from build123d import *

# Parameters (mm, degrees)
SKETCH1_R           = 2.667
BOSS_EXTRUDE1_DEPTH = 1.5875
SKETCH2_W           = 3.302
SKETCH2_H           = 18.796
CUT_EXTRUDE1_DEPTH  = 4.175


with BuildPart() as part:
    # Sketch1 → Boss-Extrude1 (new body, symmetric)
    with BuildSketch(Plane(origin=(0, 0, 0), x_dir=(0, 0, -1), z_dir=(1, 0, 0))):
        with BuildLine():
            Line((-98.171, 17.907), (94.615, 17.907))
            Line((94.615, 17.907), (94.615, 13.462))
            Line((94.615, 13.462), (98.171, 13.462))
            Line((98.171, 13.462), (98.171, 4.826))
            Line((98.171, 4.826), (94.615, 4.826))
            Line((94.615, 4.826), (94.615, 2.667))
            Line((94.615, 2.667), (89.535, 2.667))
            Line((89.535, 2.667), (89.535, 4.191))
            Line((89.535, 4.191), (83.947, 4.191))
            Line((83.947, 4.191), (83.947, 2.667))
            Line((83.947, 2.667), (76.073, 2.667))
            Line((76.073, 2.667), (76.073, -2.667))
            Line((76.073, -2.667), (83.947, -2.667))
            Line((83.947, -2.667), (83.947, -4.191))
            Line((83.947, -4.191), (89.535, -4.191))
            Line((89.535, -4.191), (89.535, -2.667))
            Line((89.535, -2.667), (94.615, -2.667))
            Line((94.615, -2.667), (94.615, -4.826))
            Line((94.615, -4.826), (98.171, -4.826))
            Line((98.171, -4.826), (98.171, -13.462))
            Line((98.171, -13.462), (94.615, -13.462))
            Line((94.615, -13.462), (94.615, -17.907))
            Line((94.615, -17.907), (-98.171, -17.907))
            Line((-98.171, -17.907), (-98.171, -6.477))
            Line((-98.171, -6.477), (-80.391, -6.477))
            ThreePointArc((-80.391, -6.477), (-73.914, 0), (-80.391, 6.477))
            Line((-80.391, 6.477), (-98.171, 6.477))
            Line((-98.171, 6.477), (-98.171, 17.907))
        make_face()
        with Locations((-63.881, 10.287)):
            Circle(SKETCH1_R, mode=Mode.SUBTRACT)
        with Locations((-63.881, -10.287)):
            Circle(SKETCH1_R, mode=Mode.SUBTRACT)
        with Locations((-44.831, 11.303)):
            Circle(SKETCH1_R, mode=Mode.SUBTRACT)
        with Locations((21.717, 11.303)):
            Circle(SKETCH1_R, mode=Mode.SUBTRACT)
        with Locations((88.265, 11.303)):
            Circle(SKETCH1_R, mode=Mode.SUBTRACT)
        with Locations((88.265, -11.303)):
            Circle(SKETCH1_R, mode=Mode.SUBTRACT)
        with Locations((21.717, -11.303)):
            Circle(SKETCH1_R, mode=Mode.SUBTRACT)
        with Locations((-44.831, -11.303)):
            Circle(SKETCH1_R, mode=Mode.SUBTRACT)
        with Locations((-9.144, 10.795)):
            Circle(SKETCH1_R, mode=Mode.SUBTRACT)
        with Locations((-32.258, 10.795)):
            Circle(SKETCH1_R, mode=Mode.SUBTRACT)
        with Locations((66.802, 10.795)):
            Circle(SKETCH1_R, mode=Mode.SUBTRACT)
        with Locations((43.688, 10.795)):
            Circle(SKETCH1_R, mode=Mode.SUBTRACT)
        with Locations((43.688, -10.795)):
            Circle(SKETCH1_R, mode=Mode.SUBTRACT)
        with Locations((66.802, -10.795)):
            Circle(SKETCH1_R, mode=Mode.SUBTRACT)
        with Locations((-32.258, -10.795)):
            Circle(SKETCH1_R, mode=Mode.SUBTRACT)
        with Locations((-9.144, -10.795)):
            Circle(SKETCH1_R, mode=Mode.SUBTRACT)
        with Locations((-20.701, 0)):
            Circle(SKETCH1_R, mode=Mode.SUBTRACT)
        with Locations((55.245, 0)):
            Circle(SKETCH1_R, mode=Mode.SUBTRACT)
    extrude(amount=BOSS_EXTRUDE1_DEPTH, both=True)

    # Sketch2 → Cut-Extrude1 (cut, through all)
    with BuildSketch(Plane(origin=(1.5875, 0, 0), x_dir=(0, 0, -1), z_dir=(1, 0, 0))):
        with Locations((-52.705, 8.509)):
            Rectangle(SKETCH2_W, SKETCH2_H)
    extrude(amount=-CUT_EXTRUDE1_DEPTH, mode=Mode.SUBTRACT)


solid = part.part
Geometry check sheet. Reference: the model listing, model coordinates, mm. A direction names the side the tool comes from. Round coordinates to 2 decimals unless told otherwise and drop trailing zeros.
Item 1: Access from +Z, -Z, +X, -X, +Y, -Y to the whole of each face (thin tool, end or side, straight path). Record for faces 4 (the flat face through (0, -6.477, 89)), 5 (the flat face through (0, 2.667, -92)), 6 (the flat face through (0, 13.462, -96)), 7 (the flat face through (0, 8, 51.054)).
Item 2: Cross-section at A-A on x = -0.15. Count the separate pieces of the cut face and the enclosed holes in it, then the cut area to 3 significant figures.
Item 3: Mould release check, pull along Y, two halves, no side actions. Record for faces 1 (the flat face through (0, 17.907, 77)), 2 (the cylindrical face through (0, 13.1, 46.8)), 3 (the flat face through (0, 8, 54.356)): pulls with the +Y half, pulls with the -Y half, needs draft (parallel to the pull), parting line crosses it, or undercut.
Item 4: Thickness scan on line 1 (Y direction, x = 0.3, z = -43.5); line 2 (Y direction, x = -0.7, z = -44); line 3 (Y direction, x = -1.1, z = 74.5). Record the ranges inside material, lowest first.
Item 5: Gauge pin test, flat ends, axial feed: pin 1 (4.5 mm diameter, centred on y = -10.795, z = -43.688, fed in from +X); pin 2 (1.7 mm diameter, centred on x = -0.5, y = -3.5, fed in from -Z) (3 decimals); pin 3 (1.6 mm diameter, centred on x = 0.5, z = -96, fed in from -Y). Record the tip position at first contact, or that the pin passes through.
Answer sheet:
1. face 4: +Z, +X, -X
1. face 5: -Z, +X, -X
1. face 6: -Z, +X, -X, +Y
1. face 7: +X, -X, +Y
2. separate pieces: 1
2. enclosed holes: 18
2. area: 6,090 mm2
3. face 1: pulls with the +Y half
3. face 2: undercut
3. face 3: needs draft
4. line 1: y = -17.91 to -13.46, -8.13 to 8.13, 13.46 to 17.91
4. line 2: y = -17.91 to -13.44, -8.15 to 8.15, 13.44 to 17.91
4. line 3: y = -17.91 to -2.69, 2.69 to 17.91
5. pin 1: passes through
5. pin 2: stops at z = -94.615
5. pin 3: stops at y = -13.46
